Check sheet for the modelled part. Datum: model origin and axes. Units: mm. A direction names the side the tool comes from. Give positions to 0.01 mm unless a question says otherwise; leave off trailing zeros. Loops run counter-clockwise (first coordinate to the right, second up) from the corner with the lowest first, then second, coordinate; pieces in that order, holes last. Notation, with made-up numbers: (73.5, -31) -> (90.5, -31) arc R25 ccw to (90.5, 1) -> close; hole circle Ø11 at (-37, -22.75). An arc over 180 degrees is marked (long way). Write each question's results on one line, items separated by ' | '. Start each with the question number.
Item 1: Mould release check, pull along X, two halves, no side actions. Record for faces 3 (the face through (24.916, 1, 88)), 4 (the face through (22.376, 1, 88)), 5 (the face through (23, 1, 177.8)): pulls with the +X half, pulls with the -X half, needs draft (parallel to the pull), parting line crosses it, or undercut.
Item 2: Cross-section at A-A on x = 11.5. Enter the section's corners in (y, z), then the cut area to 3 significant figures.
Item 3: Cross-section at B-B on y = 6.5. Enter the section's corners in (x, z).
Item 4: Cross-section at C-C on z = 123. Enter the section's corners in (x, y), then the cut area to 3 significant figures.
Item 5: Access from +Z, -Z, +X, -X, +Y, -Y to the whole of each face (thin tool, end or side, straight path). Record for faces 1 (the face through (2.056, 1, 88)), 2 (the face through (12, -11.853, 88)).
Item 6: Scan lines: line 1 along Y through (x, z) = (22, 60); line 2 along X through (y, z) = (-4.5, 92); line 3 along Y through (x, z) = (1.5, 88.9). Record each from-to range of solid material in increasing order.
from build123d import *

# Parameters (mm, degrees)
SKETCH1_W               = 25.4
SKETCH1_H               = 25.4
SKETCH1_W_2             = 20.32
SKETCH1_H_2             = 20.32
BOSS_EXTRUDE1_DEPTH     = 177.8
SKETCH2_R               = 0.5
CUT_EXTRUDE1_DEPTH      = 1
CUT_EXTRUDE1_DEPTH_BACK = 26.4
SKETCH4_R               = 0.5
CUT_EXTRUDE3_DEPTH      = 26.4


with BuildPart() as part:
    # Sketch1 → Boss-Extrude1 (new body)
    with BuildSketch(Plane.XY):
        with Locations((12.216190476, 0.846666667)):
            Rectangle(SKETCH1_W, SKETCH1_H)
        with Locations((12.216190476, 0.846666667)):
            Rectangle(SKETCH1_W_2, SKETCH1_H_2, mode=Mode.SUBTRACT)
    extrude(amount=BOSS_EXTRUDE1_DEPTH)

    # Sketch2 → Cut-Extrude1 (cut, two sides)
    with BuildSketch(Plane(origin=(24.916190476, 0, 0), x_dir=(0, 0, -1), z_dir=(1, 0, 0))) as cut_extrude1_sk:
        with Locations((-165.1, 0.846666667)):
            Circle(SKETCH2_R)
        with Locations((-152.4, 0.846666667)):
            Circle(SKETCH2_R)
        with Locations((-139.7, 0.846666667)):
            Circle(SKETCH2_R)
        with Locations((-127, 0.846666667)):
            Circle(SKETCH2_R)
        with Locations((-114.3, 0.846666667)):
            Circle(SKETCH2_R)
        with Locations((-101.6, 0.846666667)):
            Circle(SKETCH2_R)
        with Locations((-88.9, 0.846666667)):
            Circle(SKETCH2_R)
        with Locations((-76.2, 0.846666667)):
            Circle(SKETCH2_R)
        with Locations((-63.5, 0.846666667)):
            Circle(SKETCH2_R)
        with Locations((-50.8, 0.846666667)):
            Circle(SKETCH2_R)
        with Locations((-38.1, 0.846666667)):
            Circle(SKETCH2_R)
        with Locations((-25.4, 0.846666667)):
            Circle(SKETCH2_R)
        with Locations((-12.7, 0.846666667)):
            Circle(SKETCH2_R)
    extrude(amount=CUT_EXTRUDE1_DEPTH, mode=Mode.SUBTRACT)
    extrude(cut_extrude1_sk.sketch, amount=-CUT_EXTRUDE1_DEPTH_BACK, mode=Mode.SUBTRACT)

    # Sketch4 → Cut-Extrude3 (cut, through all)
    with BuildSketch(Plane(origin=(0, -11.853333333, 0), x_dir=(-1, 0, 0), z_dir=(0, -1, 0))):
        with Locations((-5.866190476, -139.7)):
            Circle(SKETCH4_R)
        with Locations((-18.566190476, -139.7)):
            Circle(SKETCH4_R)
        with Locations((-5.866190476, -114.3)):
            Circle(SKETCH4_R)
        with Locations((-18.566190476, -114.3)):
            Circle(SKETCH4_R)
    extrude(amount=-CUT_EXTRUDE3_DEPTH, mode=Mode.SUBTRACT)


solid = part.part
Answer sheet:
1) face 3: pulls with the +X half | face 4: undercut | face 5: needs draft
2) outline: (-11.85, 0) -> (-9.31, 0) -> (-9.31, 177.8) -> (-11.85, 177.8) -> close; (11.01, 0) -> (13.55, 0) -> (13.55, 177.8) -> (11.01, 177.8) -> close | area: 903 mm²
3) outline: (-0.48, 0) -> (2.06, 0) -> (2.06, 177.8) -> (-0.48, 177.8) -> close; (22.38, 0) -> (24.92, 0) -> (24.92, 177.8) -> (22.38, 177.8) -> close
4) outline: (-0.48, -11.85) -> (24.92, -11.85) -> (24.92, 13.55) -> (-0.48, 13.55) -> close; hole (2.06, -9.31) -> (22.38, -9.31) -> (22.38, 11.01) -> (2.06, 11.01) -> close | area: 232 mm²
5) face 1: +Z, -Z | face 2: +Z, -Z, +X, -X, -Y
6) line 1: y = -11.85 to -9.31, 11.01 to 13.55 | line 2: x = -0.48 to 2.06, 22.38 to 24.92 | line 3: y = -11.85 to 0.35, 1.35 to 13.55
